Geometry check sheet. Reference: drawing and pictorial views, mm from the part's lowest x, y, z. A direction names the side the tool comes from. Round coordinates to 2 decimals unless told otherwise and drop trailing zeros. Order: outer loops, then holes, each group sorted by start corner. A loop starts at its lowest first (then second) coordinate and runs counter-clockwise, first axis right, second up.
(1) Cross-section at B-B on y = 29.5. Enter the section's corners in (x, z), and give its area (3 significant figures).
(2) Gauge pin test, flat ends, axial feed: P1, Ø2, axis at y = 32, z = 20.5, coming from the +X side; P2, Ø5, axis at y = 54, z = 54.5, coming from the +X side; P3, Ø15.5, axis at x = 132.5, z = 67, coming from the -Y side. Record the tip position at first contact, or that the pin passes through.
(3) Thickness scan on L1, parallel to Z at x = 7.62, y = 3.75; L2, parallel to X at y = 10.5, z = 82.55 (1 decimal); L3, parallel to X at y = 13.75, z = 82.55 (1 decimal). Record the ranges inside material, lowest first.
(4) Set-up check for the marked faces 1, 2, 3 and 4: record each of +Z, -Z, +X, -X, +Y, -Y from which the full face is reachable in a straight line by a thin tool's end or side.
(5) Cross-section at D-D on z = 77. Enter the section's corners in (x, y), and give its area (3 significant figures).
(6) Cross-section at A-A on z = 19.05. Enter the section's corners in (x, y).
(7) Cross-section at C-C on x = 7.62. Enter the section's corners in (y, z).
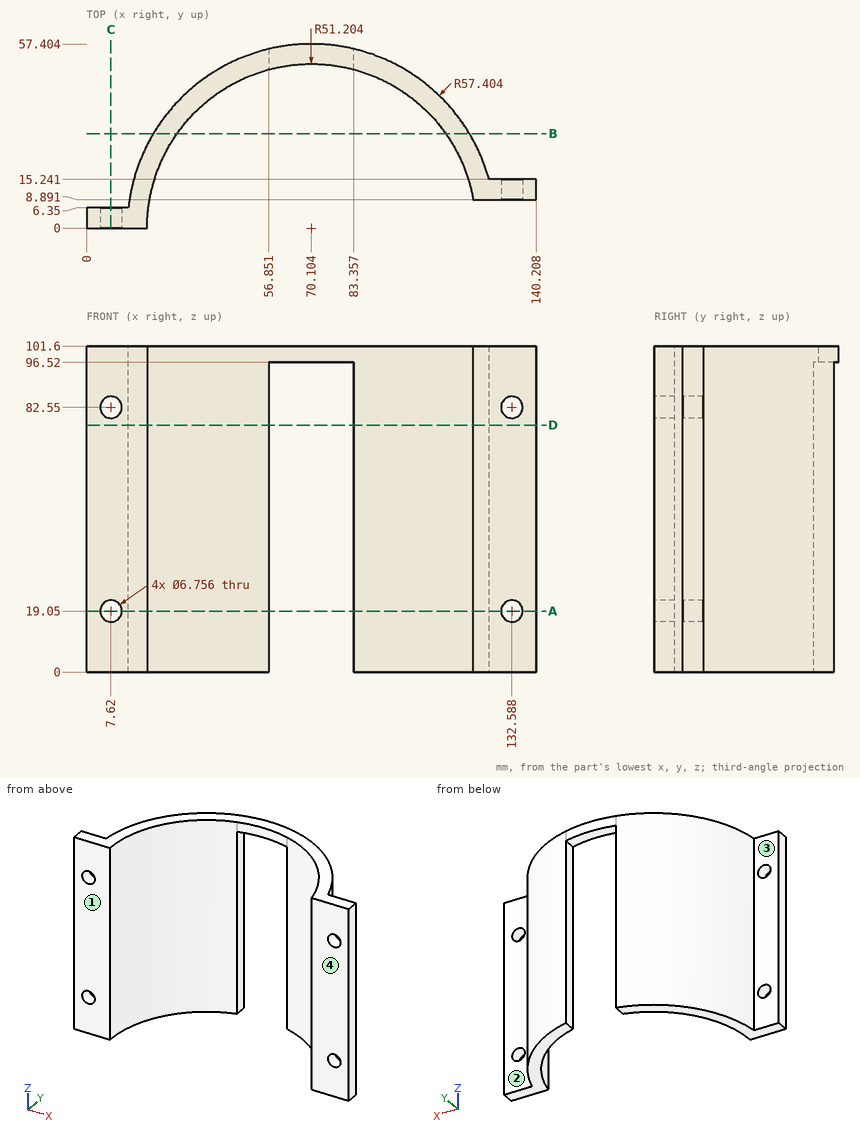
Found:
1. outline: (20.86, 0) - (28.25, 0) - (28.25, 101.6) - (20.86, 101.6) - close; (111.96, 0) - (119.35, 0) - (119.35, 101.6) - (111.96, 101.6) - close
1. area: 1,500 mm2
2. P1: stops at x = 118.42
2. P2: stops at x = 95.46
2. P3: stops at y = 8.89
3. L1: z = 0 to 15.67, 22.43 to 79.17, 85.93 to 101.6
3. L2: x = 13.7 to 20, 120.2 to 129.2, 136 to 140.2
3. L3: x = 14.4 to 20.8, 119.4 to 129.2, 136 to 140.2
4. face 1: +Z, -Z, +X, -X, -Y
4. face 2: +Z, -Z, +X, +Y
4. face 3: +Z, -Z, -X, +Y
4. face 4: +Z, -Z, +X, -Y
5. outline: (0, 0) - (18.9, 0) arc R51.2 cw to (56.85, 49.46) - (56.85, 55.85) arc R57.4 ccw to (13.05, 6.35) - (0, 6.35) - close; (83.36, 49.46) arc R51.2 cw to (120.53, 8.89) - (140.21, 8.89) - (140.21, 15.24) - (125.45, 15.24) arc R57.4 ccw to (83.36, 55.85) - close
5. area: 1,010 mm2
6. outline: (0, 0) - (4.24, 0) - (4.24, 6.35) - (0, 6.35) - close; (11, 0) - (18.9, 0) arc R51.2 cw to (56.85, 49.46) - (56.85, 55.85) arc R57.4 ccw to (13.05, 6.35) - (11, 6.35) - close; (83.36, 49.46) arc R51.2 cw to (120.53, 8.89) - (129.21, 8.89) - (129.21, 15.24) - (125.45, 15.24) arc R57.4 ccw to (83.36, 55.85) - close; (135.97, 8.89) - (140.21, 8.89) - (140.21, 15.24) - (135.97, 15.24) - close
7. outline: (0, 0) - (6.35, 0) - (6.35, 15.67) - (0, 15.67) - close; (0, 22.43) - (6.35, 22.43) - (6.35, 79.17) - (0, 79.17) - close; (0, 85.93) - (6.35, 85.93) - (6.35, 101.6) - (0, 101.6) - close
